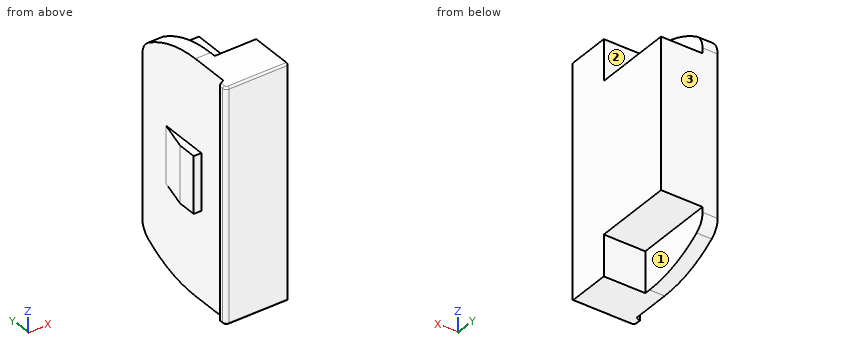
from build123d import *

# Parameters (mm, degrees)
BOSS_EXTRUDE1_DEPTH = 12.3
SKETCH2_W           = 2.2
SKETCH2_H           = 2.17
CUT_EXTRUDE1_DEPTH  = 4.2
CUT_EXTRUDE3_DEPTH  = 0.8
SKETCH5_W           = 3
SKETCH5_H           = 1
BOSS_EXTRUDE2_DEPTH = 0.4
BOSS_EXTRUDE3_DEPTH = 3
FILLET1_R           = 0.1


with BuildPart() as part:
    # Sketch1 → Boss-Extrude1 (new body)
    with BuildSketch(Plane.XY):
        with BuildLine():
            Line((0, 0), (0.299997713, 0.173208719))
            Line((0.299997713, 0.173208719), (0.299997713, 1.781598719))
            Line((0.299997713, 1.781598719), (0.299997713, 6.107458719))
            Line((0.299997713, 6.107458719), (3.299997713, 6.107458719))
            Line((3.299997713, 6.107458719), (3.299997713, 0.646828719))
            Line((3.299997713, 0.646828719), (3.299997713, -0.4))
            Line((3.299997713, -0.4), (0.2, -0.4))
            ThreePointArc((0.2, -0.4), (0.058578644, -0.341421356), (0, -0.2))
            Line((0, -0.2), (0, 0))
        make_face()
    extrude(amount=BOSS_EXTRUDE1_DEPTH)

    # Sketch2 → Cut-Extrude1 (cut)
    with BuildSketch(Plane(origin=(0, 6.107458719, 0), x_dir=(1, 0, 0), z_dir=(0, 1, 0))):
        with Locations((2.199997713, -1.085)):
            Rectangle(SKETCH2_W, SKETCH2_H)
        with Locations((2.199997713, -11.215)):
            Rectangle(SKETCH2_W, SKETCH2_H)
    extrude(amount=-CUT_EXTRUDE1_DEPTH, mode=Mode.SUBTRACT)

    # Sketch4 → Cut-Extrude3 (cut)
    with BuildSketch(Plane.ZY.offset(-0.299997713)):
        with BuildLine():
            Line((10.41158, 6.107458719), (12.3, 6.107458719))
            Line((12.3, 6.107458719), (12.3, 2.215929667))
            ThreePointArc((12.3, 2.215929667), (12.02880398, 4.022129667), (11.23913234, 5.669043272))
            ThreePointArc((11.23913234, 5.669043272), (10.879869522, 5.991150317), (10.41158, 6.107458719))
        make_face()
        with BuildLine():
            Line((1.88842, 6.107458719), (0, 6.107458719))
            Line((0, 6.107458719), (0, 2.215929667))
            ThreePointArc((0, 2.215929667), (0.27119602, 4.022129667), (1.06086766, 5.669043272))
            ThreePointArc((1.06086766, 5.669043272), (1.420130478, 5.991150317), (1.88842, 6.107458719))
        make_face()
    extrude(amount=-CUT_EXTRUDE3_DEPTH, mode=Mode.SUBTRACT)

    # Sketch5 → Boss-Extrude2 (add)
    with BuildSketch(Plane.ZY.offset(-0.299997713)):
        with Locations((6.15, 2.281598719)):
            Rectangle(SKETCH5_W, SKETCH5_H)
    extrude(amount=BOSS_EXTRUDE2_DEPTH)

    # Sketch6 → Boss-Extrude3 (add)
    with BuildSketch(Plane.XY.offset(7.65)):
        Polygon((0.299997713, 2.781598719), (0.299997713, 4.373208719), (-0.100002287, 2.781598719), align=None)
    extrude(amount=-BOSS_EXTRUDE3_DEPTH)

    # Fillet1
    fillet1_edges = [part.edges().sort_by_distance(p)[0] for p in [
        (1.749998857, -0.4, 12.3),
        (1.749998857, -0.4, 0),
        (0.058578644, -0.341421356, 0),
        (0, -0.1, 0),
        (0, -0.1, 12.3),
        (0.058578644, -0.341421356, 12.3),
    ]]
    fillet(fillet1_edges, radius=FILLET1_R)


solid = part.part
Input: part model. Units: mm. Frame: model coordinates. Face numbers are marked on the shaded views. A direction names the side the tool comes from. Give positions to 0.01 mm unless a question says otherwise; leave off trailing zeros. Loops run counter-clockwise (first coordinate to the right, second up) from the corner with the lowest first, then second, coordinate; pieces in that order, holes last. Notation, with made-up numbers: (63, 30) - (121, 30) arc R25 ccw to (121, 48) - close; hole circle Ø11 at (8, 68). An arc over 180 degrees is marked (long way). Use CSV: the item, a comma, the result in double quotes. Start each with the question number.
Item 1: Section A-A on x = 1.3. Return loops of the section in (y, z), then the cut area to 3 significant figures.
Item 2: Contact query for flat-ended pins moving along their axis: P1, Ø2, axis at y = 3.5, z = 10, coming from the -X side; P2, Ø1.5, axis at x = 1.5, y = 3.5, coming from the +Z side; P3, Ø2.5, axis at y = 3.5, z = 0.5, coming from the +X side. Output: stop coordinate, or through.
Item 3: Reachability of the marked faces 1, 2 and 3 from +Z, -Z, +X, -X, +Y, -Y: full face, straight path, thin tool, end or side. Return the list, or none.
Item 4: Line query: line 1 (X direction, y = 5, z = 2.25); line 2 (Z direction, x = 3.05, y = 3.5); line 3 (X direction, y = 2, z = 1.5). Output: solid intervals per line, ascending.
Item 5: Section D-D on x = 0.55. Return loops of the section in (y, z).
Item 6: Section C-C on y = 3. Return loops of the section in (x, z).
Item 7: Section B-B on z = 5. Return loops of the section in (x, y), then the cut area to 3 significant figures.
Ans:
1,outline,"(-0.4, 0.1) arc R0.1 ccw to (-0.3, 0) - (1.91, 0) - (1.91, 2.17) - (6.11, 2.17) - (6.11, 10.13) - (1.91, 10.13) - (1.91, 12.3) - (-0.3, 12.3) arc R0.1 ccw to (-0.4, 12.2) - close"
1,area,"61.8 mm2"
2,P1,"stops at x = 0.3"
2,P2,"stops at z = 12.27"
2,P3,"stops at x = 1.1"
3,face 1,"-Z, +X, +Y"
3,face 2,"+Z, +X, +Y"
3,face 3,"+Z, -Z, +X, -X, +Y"
4,line 1,"x = 0.3 to 3.3"
4,line 2,"z = 2.17 to 10.13"
4,line 3,"x = 0.3 to 1.1"
5,outline,"(-0.4, 0.1) arc R0.1 ccw to (-0.3, 0) - (2.22, 0) arc R6.15 ccw to (5.67, 1.06) arc R1 ccw to (6.11, 1.89) - (6.11, 10.41) arc R1 ccw to (5.67, 11.24) arc R6.15 ccw to (2.22, 12.3) - (-0.3, 12.3) arc R0.1 ccw to (-0.4, 12.2) - close"
6,outline,"(-0.05, 4.65) - (0.3, 4.65) - (0.3, 0.05) - (1.1, 0.05) - (1.1, 2.17) - (3.3, 2.17) - (3.3, 10.13) - (1.1, 10.13) - (1.1, 12.25) - (0.3, 12.25) - (0.3, 7.65) - (-0.05, 7.65) - close"
7,outline,"(-0.1, 1.78) - (0.3, 1.78) - (0.3, 0.17) - (0, 0) - (0, -0.2) arc R0.2 ccw to (0.2, -0.4) - (3.3, -0.4) - (3.3, 6.11) - (0.3, 6.11) - (0.3, 4.37) - (-0.1, 2.78) - close"
7,area,"20.4 mm2"
